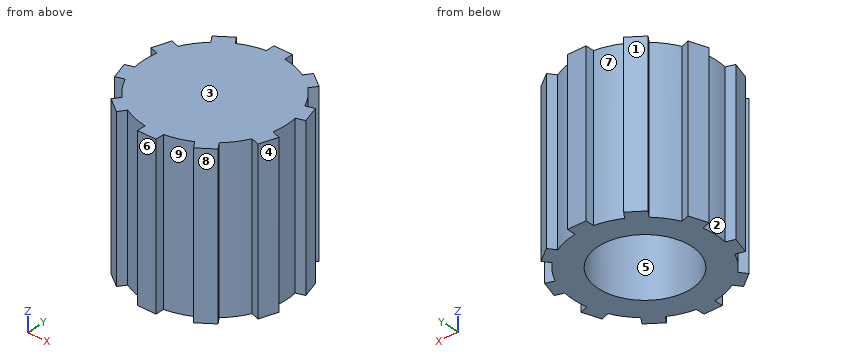
Autodesk Inventor part; units mm, degrees
ref_plane "Work Plane2" through (0, 0, 29) normal (0, 0, 1) x (1, 0, 0)
ref_plane "YZ Plane" through (0, 0, 0) normal (1, 0, 0) x (0, 1, 0)
ref_plane "XZ Plane" through (0, 0, 0) normal (0, 1, 0) x (-1, 0, 0)
sketch "Sketch1" plane through (0, 0, 0) normal (0, 0, 1) x (1, 0, 0)
  circle A0 centre (0, 0) radius 17 construction
  circle A1 centre (0, 0) radius 8.5
  line L0 (-1.727, 14.5) -> (1.69, 14.5)
  line L1 (1.69, 14.5) -> (1.69, 12.8897)
  line L2 (-1.727, 12.8848) -> (-1.727, 14.5)
  line L3 (-7.1557, 12.7241) -> (-6.2091, 11.4213)
  line L4 (-9.92, 10.7157) -> (-7.1557, 12.7241)
  line L5 (-8.9706, 9.4089) -> (-9.92, 10.7157)
  line L6 (-13.2681, 6.088) -> (-11.7366, 5.5904)
  line L7 (-14.324, 2.8383) -> (-13.2681, 6.088)
  line L8 (-12.7878, 2.3392) -> (-14.324, 2.8383)
  line L9 (-14.3126, -2.8735) -> (-12.7811, -2.3759)
  line L10 (-13.2567, -6.1232) -> (-14.3126, -2.8735)
  line L11 (-11.7205, -5.624) -> (-13.2567, -6.1232)
  line L12 (-9.8901, -10.7374) -> (-8.9436, -9.4346)
  line L13 (-7.1258, -12.7458) -> (-9.8901, -10.7374)
  line L14 (-6.1764, -11.4391) -> (-7.1258, -12.7458)
  line L15 (-1.69, -14.5) -> (-1.69, -12.8897)
  line L16 (1.727, -14.5) -> (-1.69, -14.5)
  line L17 (1.727, -12.8848) -> (1.727, -14.5)
  line L18 (7.1557, -12.7241) -> (6.2091, -11.4213)
  line L19 (9.92, -10.7157) -> (7.1557, -12.7241)
  line L20 (8.9706, -9.4089) -> (9.92, -10.7157)
  line L21 (13.2681, -6.088) -> (11.7366, -5.5904)
  line L22 (14.324, -2.8383) -> (13.2681, -6.088)
  line L23 (12.7878, -2.3392) -> (14.324, -2.8383)
  line L24 (14.3126, 2.8735) -> (12.7811, 2.3759)
  line L25 (13.2567, 6.1232) -> (14.3126, 2.8735)
  line L26 (11.7205, 5.624) -> (13.2567, 6.1232)
  line L27 (9.8901, 10.7374) -> (8.9436, 9.4346)
  line L28 (7.1258, 12.7458) -> (9.8901, 10.7374)
  line L29 (6.1764, 11.4391) -> (7.1258, 12.7458)
  arc A2 (-1.727, 12.8848) -> (-6.2091, 11.4213) centre (0, 0) ccw construction
  arc A3 (-1.727, 12.8848) -> (-6.2091, 11.4213) centre (0, 0) ccw
  arc A4 (-8.9706, 9.4089) -> (-11.7366, 5.5904) centre (0, 0) ccw
  arc A5 (-8.9706, 9.4089) -> (-11.7366, 5.5904) centre (0, 0) ccw construction
  arc A6 (-12.7878, 2.3392) -> (-12.7811, -2.3759) centre (0, 0) ccw
  arc A7 (-12.7878, 2.3392) -> (-12.7811, -2.3759) centre (0, 0) ccw construction
  arc A8 (-11.7205, -5.624) -> (-8.9436, -9.4346) centre (0, 0) ccw
  arc A9 (-11.7205, -5.624) -> (-8.9436, -9.4346) centre (0, 0) ccw construction
  arc A10 (6.1764, 11.4391) -> (1.69, 12.8897) centre (0, 0) ccw construction
  arc A11 (6.1764, 11.4391) -> (1.69, 12.8897) centre (0, 0) ccw
  arc A12 (12.7878, -2.3392) -> (12.7811, 2.3759) centre (0, 0) ccw
  arc A13 (12.7878, -2.3392) -> (12.7811, 2.3759) centre (0, 0) ccw construction
  arc A14 (8.9706, -9.4089) -> (11.7366, -5.5904) centre (0, 0) ccw
  arc A15 (8.9706, -9.4089) -> (11.7366, -5.5904) centre (0, 0) ccw construction
  arc A16 (-6.1764, -11.4391) -> (-1.69, -12.8897) centre (0, 0) ccw
  arc A17 (1.727, -12.8848) -> (6.2091, -11.4213) centre (0, 0) ccw
  arc A18 (-6.1764, -11.4391) -> (-1.69, -12.8897) centre (0, 0) ccw construction
  arc A19 (1.727, -12.8848) -> (6.2091, -11.4213) centre (0, 0) ccw construction
  arc A20 (11.7205, 5.624) -> (8.9436, 9.4346) centre (0, 0) ccw
  dimension "d5" = 360
  dimension "d14" = 6
  dimension "d15" = 13
  dimension "d16" = 34
  dimension "d17" = 17
extrude "Extrusion1" add sketch "Sketch1" along normal blind 29
sketch "Sketch2" plane through (0, 0, 29) normal (0, 0, 1) x (1, 0, 0)
  line L0 (-6.2091, 11.4213) -> (-7.1557, 12.7241)
  line L1 (-7.1557, 12.7241) -> (-9.92, 10.7157)
  line L2 (-9.92, 10.7157) -> (-8.9706, 9.4089)
  arc A0 (-8.9706, 9.4089) -> (-11.7366, 5.5904) centre (0, 0) ccw
  line L3 (-11.7366, 5.5904) -> (-13.2681, 6.088)
  line L4 (-13.2681, 6.088) -> (-14.324, 2.8383)
  line L5 (-14.324, 2.8383) -> (-12.7878, 2.3392)
  arc A1 (-12.7878, 2.3392) -> (-12.7811, -2.3759) centre (0, 0) ccw
  line L6 (-12.7811, -2.3759) -> (-14.3126, -2.8735)
  line L7 (-14.3126, -2.8735) -> (-13.2567, -6.1232)
  line L8 (-13.2567, -6.1232) -> (-11.7205, -5.624)
  arc A2 (-11.7205, -5.624) -> (-8.9436, -9.4346) centre (0, 0) ccw
  line L9 (-8.9436, -9.4346) -> (-9.8901, -10.7374)
  line L10 (-9.8901, -10.7374) -> (-7.1258, -12.7458)
  line L11 (-7.1258, -12.7458) -> (-6.1764, -11.4391)
  arc A3 (-6.1764, -11.4391) -> (-1.69, -12.8897) centre (0, 0) ccw
  line L12 (-1.69, -12.8897) -> (-1.69, -14.5)
  line L13 (-1.69, -14.5) -> (1.727, -14.5)
  line L14 (1.727, -14.5) -> (1.727, -12.8848)
  arc A4 (1.727, -12.8848) -> (6.2091, -11.4213) centre (0, 0) ccw
  line L15 (6.2091, -11.4213) -> (7.1557, -12.7241)
  line L16 (7.1557, -12.7241) -> (9.92, -10.7157)
  line L17 (9.92, -10.7157) -> (8.9706, -9.4089)
  arc A5 (8.9706, -9.4089) -> (11.7366, -5.5904) centre (0, 0) ccw
  line L18 (11.7366, -5.5904) -> (13.2681, -6.088)
  line L19 (13.2681, -6.088) -> (14.324, -2.8383)
  line L20 (14.324, -2.8383) -> (12.7878, -2.3392)
  arc A6 (12.7878, -2.3392) -> (12.7811, 2.3759) centre (0, 0) ccw
  line L21 (12.7811, 2.3759) -> (14.3126, 2.8735)
  line L22 (14.3126, 2.8735) -> (13.2567, 6.1232)
  line L23 (13.2567, 6.1232) -> (11.7205, 5.624)
  arc A7 (11.7205, 5.624) -> (8.9436, 9.4346) centre (0, 0) ccw
  line L24 (8.9436, 9.4346) -> (9.8901, 10.7374)
  line L25 (9.8901, 10.7374) -> (7.1258, 12.7458)
  line L26 (7.1258, 12.7458) -> (6.1764, 11.4391)
  arc A8 (6.1764, 11.4391) -> (1.69, 12.8897) centre (0, 0) ccw
  line L27 (1.69, 12.8897) -> (1.69, 14.5)
  line L28 (1.69, 14.5) -> (-1.727, 14.5)
  line L29 (-1.727, 14.5) -> (-1.727, 12.8848)
  arc A9 (-1.727, 12.8848) -> (-6.2091, 11.4213) centre (0, 0) ccw
  circle A10 centre (0, 0) radius 8.5
  circle A11 centre (0, 0) radius 8.5
extrude "Extrusion2" add sketch "Sketch2" against normal blind 11 contours A10
sketch "Sketch3" plane through (0, 0, 18) normal (0, 0, -1) x (-1, 0, 0)
  arc A0 (1.3217, 0.7094) -> (0.5581, -1.3923) centre (0, 0) ccw
  line L0 (0.5581, -1.3923) -> (1.3217, 0.7094)
  circle A1 centre (0, 0) radius 2.5
  point P0 (0, 0)
  dimension "d11" = 5
extrude "Extrusion3" add sketch "Sketch3" along normal blind 9
ref_plane "Work Plane1" through (-0.5337, -1.6424, 0) normal (-0.9511, 0.309, 0) x (0, 0, 1)
sketch "Sketch4" plane through (-0.5337, -1.6424, 0) normal (-0.9511, 0.309, 0) x (0, 0, 1)
  line L0 (31.9338, 1.727) -> (-3.3978, 1.727) construction
  point P0 (0, 1.727)
ref_plane "Work Plane2" through (0, 0, 29) normal (0, 0, 1) x (1, 0, 0)
sketch "Sketch5" plane through (0, 0, 29) normal (0, 0, 1) x (1, 0, 0)
  circle A0 centre (0, 0) radius 17 construction
  dimension "d19" = 34
properties part number "felga_CPY"
CAD build for the part. Positions are in the model's coordinates, mm. Face numbers are marked on the shaded views. A direction names the side the tool comes from. Give positions to 0.01 mm unless a question says otherwise; leave off trailing zeros. Order: outer loops, then holes, each group sorted by start corner. A loop starts at its lowest first (then second) coordinate and runs counter-clockwise, first axis right, second up. Notation, with made-up numbers: M 1.25,58 L 37.25,58 A16 ccw 37.25,84 Z; hole C 66.5,-34 d3. An arc over 180 degrees is marked long. Put each result on its own line as item: value. Start each with the question number.
(1) Drill centre lines: line 1 along Z through (x, y) = (6, 1.5); line 2 along Y through (x, z) = (-6, 17.5); line 3 along Y through (x, z) = (0, 6.5). Where is each one in solid material? Low to high.
(2) Which spindle directions (+Z, -Z, +X, -X, +Y, -Y) get a long thin tool onto all of the face, cutting with end or side? Do the marked faces 5, 6, 7, 8 and 9. Say none if no direction does.
(3) Saw through at A-A, the plane z = 13.5. Give the number of separate pieces and of enclosed holes in the cut face, then the cut area to 3 significant figures.
(4) Flat gauge pins, fed straight in: pin 1 Ø6 at (y, z) = (5.5, 6.5) entering from -X; pin 2 Ø1.4 at (x, y) = (0.5, -0.5) entering from -Z; pin 3 Ø0.8 at (y, z) = (-13.5, 19.5) entering from -X. Where does each tip first touch, or does it go through?
(5) Saw through at C-C, the plane y = 0. Write the cut outline in (x, z), then the cut area to 3 significant figures.
(6) Saw through at D-D, the plane y = -3.5. Write the cut outline in (x, z).
(7) Mould opens along Y. For the marked faces 1, 2, 3 and 4 say: +Y half, -Y half, draft (parallel to the pull), parting line (faces both ways), or undercut.
(8) Saw through at B-B, the plane x = 0. Write the cut outline in (y, z).
Check result:
1. line 1: z = 18 to 29
1. line 2: y = -11.53 to -6.02, 6.02 to 11.53
1. line 3: y = -14.5 to -8.5, 8.5 to 14.5
2. face 5: -Z
2. face 6: +Z, -Z, +X, -X, -Y
2. face 7: +Z, -Z, +Y
2. face 8: +Z, -Z, +X, -Y
2. face 9: +Z, -Z, -Y
3. separate pieces: 2
3. enclosed holes: 2
3. area: 370 mm2
4. pin 1: stops at x = -14.32
4. pin 2: stops at z = 18
4. pin 3: stops at x = -1.69
5. outline: M -13,0 L -8.5,0 L -8.5,18 L -2.5,18 L -2.5,9 L -1.06,9 L -1.06,18 L 1.5,18 L 1.5,9 L 2.5,9 L 2.5,18 L 8.5,18 L 8.5,0 L 13,0 L 13,29 L -13,29 Z
5. area: 470 mm2
6. outline: M -14.11,0 L -7.75,0 L -7.75,18 L 7.75,18 L 7.75,0 L 14.11,0 L 14.11,29 L -14.11,29 Z
7. face 1: +Y half
7. face 2: undercut
7. face 3: draft
7. face 4: -Y half
8. outline: M -14.5,0 L -8.5,0 L -8.5,18 L -2.5,18 L -2.5,9 L -1.5,9 L -1.5,18 L 1.5,18 L 1.5,9 L 2.5,9 L 2.5,18 L 8.5,18 L 8.5,0 L 14.5,0 L 14.5,29 L -14.5,29 Z
